Source: CAD feature listing. Evaluate the final solid. Frame: model axes, mm. Give positions to 0.01 mm unless a question says otherwise; leave off trailing zeros. Order: outer loops, then holes, each group sorted by start corner. A loop starts at its lowest first (then second) coordinate and runs counter-clockwise, first axis right, second up. Notation, with made-up numbers: (41.25, -38) - (98.25, -38) arc R14 ccw to (98.25, -14) - close; hole circle Ø9 at (-23.5, 43). An arc over 180 degrees is marked (long way). Write each question's results on one line, items separated by ' | '. Start each with the question number.
Item 1: Section A-A on x = 62.23. Output: boundary loops of the cut face in (y, z).
Item 2: Line query: line 1 along Z through (x, y) = (62.23, 2.35); line 2 along Y through (x, z) = (64.5, -32); line 3 along Y through (x, z) = (73, -75). Output: solid intervals per line, ascending.
Item 3: Section B-B on z = -13.97. Output: boundary loops of the cut face in (x, y) (3 decimals).
Item 4: Section C-C on z = -32. Output: boundary loops of the cut face in (x, y) (3 decimals), and give its area (3 significant figures).
Item 5: Contact query for flat-ended pins moving along their axis: pin 1 Ø4.5 at (x, z) = (62.23, -13.97) entering from -Y; pin 2 Ø1.8 at (x, y) = (72, 18) entering from -Z; pin 3 Ø4.5 at (x, z) = (62.23, -74.93) entering from +Y; pin 4 Ø7 at (x, z) = (68.5, -102.5) entering from +Y. Output: stop coordinate, or through.
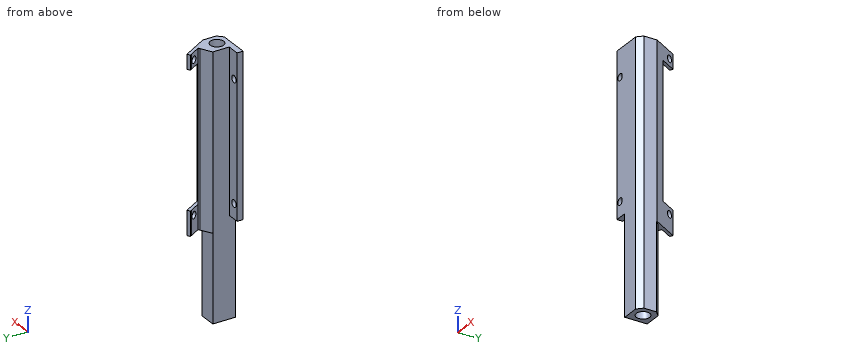
```python
from build123d import *

# Parameters (mm, degrees)
SKETCH1_W           = 77.47
SKETCH1_H           = 133.35
BOSS_EXTRUDE1_DEPTH = 11.43
SKETCH2_R           = 3.429
CUT_EXTRUDE1_DEPTH  = 134.35
CUT_EXTRUDE2_DEPTH  = 12.43
SKETCH4_W           = 54.61
SKETCH4_H           = 6.35
CUT_EXTRUDE3_DEPTH  = 134.35
CHAMFER1_SIZE       = 2.54
SKETCH5_W           = 66.04
SKETCH5_H           = 50.8
CUT_EXTRUDE4_DEPTH  = 12.43
SKETCH6_W           = 53.34
SKETCH6_H           = 82.55
CUT_EXTRUDE5_DEPTH  = 12.43
SKETCH7_R           = 1.778
HOLE_CUTS_1_DEPTH   = 6.08
BOSS_EXTRUDE2_DEPTH = 88.9
CUT_EXTRUDE7_REACH  = 135.35
SKETCH9_W           = 6.35
SKETCH9_H           = 5.08
CUT_EXTRUDE8_REACH  = 135.35
SKETCH10_W          = 6.35
SKETCH10_H          = 1.27
HOLE_CUTS_2_REACH   = 10.608
SKETCH11_R          = 1.778
SKETCH12_W          = 88.9
SKETCH12_H          = 11.176
CUT_EXTRUDE10_DEPTH = 1.27
CUT_EXTRUDE15_DEPTH = 134.35
SKETCH14_W          = 6.35
SKETCH14_H          = 82.55
CUT_EXTRUDE12_DEPTH = 0.762
SKETCH15_W          = 1.676805635
SKETCH15_H          = 88.9
BOSS_EXTRUDE3_DEPTH = 1.27
CUT_EXTRUDE13_REACH = 10.019
SKETCH16_W          = 69.088
SKETCH16_H          = 9.3345
CUT_EXTRUDE14_REACH = 12.28
SKETCH17_W          = 1.27
SKETCH17_H          = 88.9


with BuildPart() as part:
    # Sketch1 → Boss-Extrude1 (new body)
    with BuildSketch(Plane(origin=(0, 0, 0), x_dir=(1, 0, 0), z_dir=(0, 1, 0))):
        with Locations((38.735, 66.675)):
            Rectangle(SKETCH1_W, SKETCH1_H)
    extrude(amount=BOSS_EXTRUDE1_DEPTH)

    # Sketch2 → Cut-Extrude1 (cut, through all)
    with BuildSketch(Plane.XY):
        with Locations((5.715, 5.715)):
            Circle(SKETCH2_R)
        with Locations((71.755, 5.715)):
            Circle(SKETCH2_R)
    extrude(amount=-CUT_EXTRUDE1_DEPTH, mode=Mode.SUBTRACT)

    # Sketch3 → Cut-Extrude2 (cut, through all)
    with BuildSketch(Plane(origin=(0, 11.43, 0), x_dir=(1, 0, 0), z_dir=(0, 1, 0))):
        with BuildLine():
            Line((11.43, 133.35), (11.43, 95.25))
            ThreePointArc((11.43, 95.25), (15.149743879, 86.269743879), (24.13, 82.55))
            Line((24.13, 82.55), (53.34, 82.55))
            ThreePointArc((53.34, 82.55), (62.320256121, 86.269743879), (66.04, 95.25))
            Line((66.04, 95.25), (66.04, 133.35))
            Line((66.04, 133.35), (11.43, 133.35))
        make_face()
    extrude(amount=-CUT_EXTRUDE2_DEPTH, mode=Mode.SUBTRACT)

    # Sketch4 → Cut-Extrude3 (cut, through all)
    with BuildSketch(Plane(origin=(0, 0, -133.35), x_dir=(-1, 0, 0), z_dir=(0, 0, -1))):
        with Locations((-38.735, 8.255)):
            Rectangle(SKETCH4_W, SKETCH4_H)
    extrude(amount=-CUT_EXTRUDE3_DEPTH, mode=Mode.SUBTRACT)

    # Chamfer1
    chamfer1_edges = [part.edges().sort_by_distance(p)[0] for p in [
        (77.47, 11.43, -66.675),
        (0, 11.43, -66.675),
        (77.47, 0, -66.675),
        (0, 0, -66.675),
    ]]
    chamfer(chamfer1_edges, length=CHAMFER1_SIZE)

    # Sketch5 → Cut-Extrude4 (cut, through all)
    with BuildSketch(Plane(origin=(0, 11.43, 0), x_dir=(1, 0, 0), z_dir=(0, 1, 0))):
        with Locations((33.02, 107.95)):
            Rectangle(SKETCH5_W, SKETCH5_H)
    extrude(amount=-CUT_EXTRUDE4_DEPTH, mode=Mode.SUBTRACT)

    # Sketch6 → Cut-Extrude5 (cut, through all)
    with BuildSketch(Plane(origin=(0, 11.43, 0), x_dir=(1, 0, 0), z_dir=(0, 1, 0))):
        with Locations((26.67, 41.275)):
            Rectangle(SKETCH6_W, SKETCH6_H)
    extrude(amount=-CUT_EXTRUDE5_DEPTH, mode=Mode.SUBTRACT)

    # Sketch7 → Hole Cuts 1 (cut, through all)
    with BuildSketch(Plane(origin=(0, 5.08, 0), x_dir=(1, 0, 0), z_dir=(0, 1, 0))):
        with Locations((62.23, 74.93)):
            Circle(SKETCH7_R)
        with Locations((62.23, 13.97)):
            Circle(SKETCH7_R)
    extrude(amount=-HOLE_CUTS_1_DEPTH, mode=Mode.SUBTRACT)

    # Sketch8 → Boss-Extrude2 (add)
    with BuildSketch(Plane.XY):
        Polygon((77.47, 11.869940905), (77.47, 8.89), (74.93, 11.43), (66.04, 11.43), (71.539261314, 14.605), (68.618261314, 19.664320409), (71.882, 21.548640818), align=None)
    extrude(amount=-BOSS_EXTRUDE2_DEPTH)

    # Sketch9 → Cut-Extrude7 (cut, up to next)
    with BuildSketch(Plane.XY, mode=Mode.PRIVATE) as cut_extrude7_sk1:
        with Locations((56.515, 2.54)):
            Rectangle(SKETCH9_W, SKETCH9_H)
    cut_extrude7_tool1 = extrude(cut_extrude7_sk1.sketch, amount=-CUT_EXTRUDE7_REACH, mode=Mode.PRIVATE) & part.part
    add(cut_extrude7_tool1.solids().sort_by_distance((56.515, 2.54, 0))[0], mode=Mode.SUBTRACT)

    # Sketch10 → Cut-Extrude8 (cut, up to next)
    with BuildSketch(Plane.XY, mode=Mode.PRIVATE) as cut_extrude8_sk1:
        with Locations((62.865, 4.445)):
            Rectangle(SKETCH10_W, SKETCH10_H)
    cut_extrude8_tool1 = extrude(cut_extrude8_sk1.sketch, amount=-CUT_EXTRUDE8_REACH, mode=Mode.PRIVATE) & part.part
    add(cut_extrude8_tool1.solids().sort_by_distance((62.865, 4.445, 0))[0], mode=Mode.SUBTRACT)

    # Sketch11 → Hole Cuts 2 (cut, up to next)
    with BuildSketch(Plane(origin=(59.978596497, 34.628658833, 0), x_dir=(0, 0, 1), z_dir=(-0.866025404, -0.5, 0)), mode=Mode.PRIVATE) as hole_cuts_2_sk1:
        with Locations((-3.81, -19.311329635)):
            Circle(SKETCH11_R)
    hole_cuts_2_tool1 = extrude(hole_cuts_2_sk1.sketch, amount=-HOLE_CUTS_2_REACH, mode=Mode.PRIVATE) & part.part
    add(hole_cuts_2_tool1.solids().sort_by_distance((69.634261, 17.904557, -3.81))[0], mode=Mode.SUBTRACT)
    # Sketch11 → Hole Cuts 2 (cut, up to next)
    with BuildSketch(Plane(origin=(59.978596497, 34.628658833, 0), x_dir=(0, 0, 1), z_dir=(-0.866025404, -0.5, 0)), mode=Mode.PRIVATE) as hole_cuts_2_sk2:
        with Locations((-80.01, -19.311329635)):
            Circle(SKETCH11_R)
    hole_cuts_2_tool2 = extrude(hole_cuts_2_sk2.sketch, amount=-HOLE_CUTS_2_REACH, mode=Mode.PRIVATE) & part.part
    add(hole_cuts_2_tool2.solids().sort_by_distance((69.634261, 17.904557, -80.01))[0], mode=Mode.SUBTRACT)

    # Sketch12 → Cut-Extrude10 (cut)
    with BuildSketch(Plane(origin=(63.242335183, 36.512979242, 0), x_dir=(0, 0, -1), z_dir=(0.866025404, 0.5, 0))):
        with Locations((44.45, -22.867329635)):
            Rectangle(SKETCH12_W, SKETCH12_H)
    extrude(amount=-CUT_EXTRUDE10_DEPTH, mode=Mode.SUBTRACT)

    # Sketch22 → Cut-Extrude15 (cut, through all)
    with BuildSketch(Plane.XY):
        Polygon((64.930582409, 17.535238), (69.32999146, 20.075238), (72.25099146, 15.015917591), (67.851582409, 12.475917591), align=None)
    extrude(amount=-CUT_EXTRUDE15_DEPTH, mode=Mode.SUBTRACT)

    # Sketch14 → Cut-Extrude12 (cut)
    with BuildSketch(Plane(origin=(0, 3.81, 0), x_dir=(1, 0, 0), z_dir=(0, 1, 0))):
        with Locations((62.865, 41.275)):
            Rectangle(SKETCH14_W, SKETCH14_H)
    extrude(amount=-CUT_EXTRUDE12_DEPTH, mode=Mode.SUBTRACT)

    # Sketch15 → Boss-Extrude3 (add)
    with BuildSketch(Plane(origin=(8.639664817, -14.964338424, 0), x_dir=(0.866025404, 0.5, 0), z_dir=(-0.5, 0.866025404, 0))):
        with Locations((70.917555667, 44.45)):
            Rectangle(SKETCH15_W, SKETCH15_H)
    extrude(amount=BOSS_EXTRUDE3_DEPTH)

    # Sketch16 → Cut-Extrude13 (cut, up to next)
    with BuildSketch(Plane(origin=(60.690326643, 35.039576424, 0), x_dir=(0, 0, 1), z_dir=(-0.866025404, -0.5, 0)), mode=Mode.PRIVATE) as cut_extrude13_sk1:
        with Locations((-41.91, -20.676579635)):
            Rectangle(SKETCH16_W, SKETCH16_H)
    cut_extrude13_tool1 = extrude(cut_extrude13_sk1.sketch, amount=-CUT_EXTRUDE13_REACH, mode=Mode.PRIVATE) & part.part
    add(cut_extrude13_tool1.solids().sort_by_distance((71.028616, 17.133133, -41.91))[0], mode=Mode.SUBTRACT)

    # Sketch17 → Cut-Extrude14 (cut, up to next)
    with BuildSketch(Plane(origin=(14.227664817, -24.643038337, 0), x_dir=(0.866025404, 0.5, 0), z_dir=(-0.5, 0.866025404, 0)), mode=Mode.PRIVATE) as cut_extrude14_sk1:
        with Locations((72.390958484, 44.45)):
            Rectangle(SKETCH17_W, SKETCH17_H)
    cut_extrude14_tool1 = extrude(cut_extrude14_sk1.sketch, amount=-CUT_EXTRUDE14_REACH, mode=Mode.PRIVATE) & part.part
    add(cut_extrude14_tool1.solids().sort_by_distance((76.920074, 11.552441, -44.45))[0], mode=Mode.SUBTRACT)


solid = part.part
```
Evaluation:
1) outline: (0, -82.55) - (3.05, -82.55) - (3.05, -76.71) - (0, -76.71) - close; (0, -73.15) - (3.05, -73.15) - (3.05, -15.75) - (0, -15.75) - close; (0, -12.19) - (3.05, -12.19) - (3.05, 0) - (0, 0) - close
2) line 1: z = -82.55 to -76.71, -73.15 to -15.75, -12.19 to 0 | line 2: y = 0 to 3.05 | line 3: y = 0 to 2.52, 8.91 to 13.72
3) outline: (59.69, 0) - (60.452, 0) - (60.452, 3.048) - (59.69, 3.048) - close; (64.008, 0) - (74.93, 0) - (77.47, 2.54) - (77.47, 9.33) - (74.814, 13.93) - (73.362, 13.091) - (72.251, 15.016) - (66.04, 11.43) - (66.04, 3.048) - (64.008, 3.048) - close; hole circle Ø6.858 at (71.755, 5.715)
4) outline: (59.69, 0) - (74.93, 0) - (77.47, 2.54) - (77.47, 9.33) - (74.814, 13.93) - (73.362, 13.091) - (72.251, 15.016) - (66.04, 11.43) - (66.04, 3.048) - (59.69, 3.048) - close; hole circle Ø6.858 at (71.755, 5.715) | area: 127 mm^2
5) pin 1: stops at y = 0 | pin 2: stops at z = -88.9 | pin 3: stops at y = 3.05 | pin 4: stops at y = 11.43
